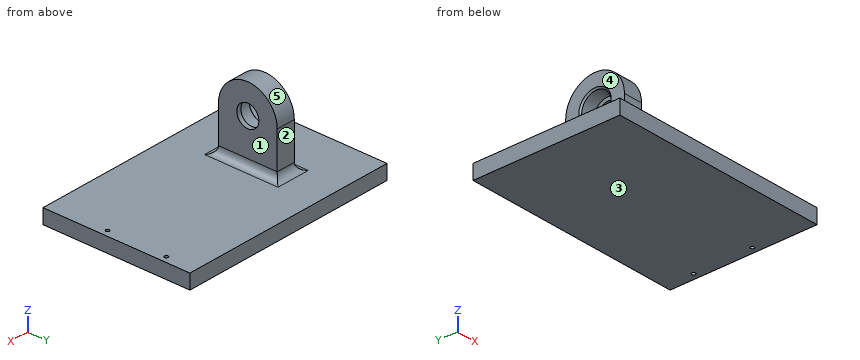
from build123d import *

# Parameters (mm, degrees)
SKETCH_2_W          = 150
SKETCH_2_H          = 100
EXTRUDE_1_DEPTH     = 10
SKETCH_3_W          = 13
SKETCH_3_H          = 40
EXTRUDE_2_DEPTH     = 40
SKETCH_4_R          = 20
EXTRUDE_3_DEPTH     = 13
SKETCH_5_R          = 10
CUT_EXTRUDE_1_DEPTH = 10
M3X0_5_2_D          = 2.5
FILLET_1_R          = 5
SKETCH_12_R         = 7.5
CUT_EXTRUDE_2_DEPTH = 130.263297188
CHAMFER_1_SIZE      = 1


with BuildPart() as part:
    # ｽｹｯﾁ2 → ﾎﾞｽ - 押し出し1 (new body)
    with BuildSketch(Plane.XY):
        Rectangle(SKETCH_2_W, SKETCH_2_H)
    extrude(amount=EXTRUDE_1_DEPTH)

    # ｽｹｯﾁ3 → ﾎﾞｽ - 押し出し2 (add)
    with BuildSketch(Plane.XY):
        with Locations((-31.5, 0)):
            Rectangle(SKETCH_3_W, SKETCH_3_H)
    extrude(amount=EXTRUDE_2_DEPTH)

    # ｽｹｯﾁ4 → ﾎﾞｽ - 押し出し3 (add)
    with BuildSketch(Plane.ZY.offset(38)):
        with Locations((40, 0)):
            Circle(SKETCH_4_R)
    extrude(amount=-EXTRUDE_3_DEPTH)

    # ｽｹｯﾁ5 → ｶｯﾄ - 押し出し1 (cut)
    with BuildSketch(Plane.ZY.offset(38)):
        with Locations(Location((40, 0, 0), (0, 0, 270))):
            Circle(SKETCH_5_R)
    extrude(amount=-CUT_EXTRUDE_1_DEPTH, mode=Mode.SUBTRACT)

    # M3x0.5 ねじ穴2 (through all)
    with Locations(Plane.XY.offset(10)):
        with Locations((70.5, -10.000898701), (70.5, 29.999101299)):
            Hole(M3X0_5_2_D / 2)

    # ﾌｨﾚｯﾄ1
    fillet_1_edges = [part.edges().sort_by_distance(p)[0] for p in [
        (-31.5, 20, 10),
        (-38, 0, 10),
        (-31.5, -20, 10),
        (-25, 0, 10),
    ]]
    fillet(fillet_1_edges, radius=FILLET_1_R)

    # ｽｹｯﾁ12 → ｶｯﾄ - 押し出し2 (cut, through all)
    with BuildSketch(Plane.ZY.offset(28)):
        with Locations(Location((40, 0, 0), (0, 0, 270))):
            Circle(SKETCH_12_R)
    extrude(amount=-CUT_EXTRUDE_2_DEPTH, mode=Mode.SUBTRACT)

    # 面取り1
    chamfer_1_edges = [part.edges().sort_by_distance(p)[0] for p in [
        (-38, 10, 40),
    ]]
    chamfer(chamfer_1_edges, length=CHAMFER_1_SIZE)


solid = part.part
Verification items for the finished model (mm, model axes). Face numbers are marked on the shaded views. A direction names the side the tool comes from. Coordinates: 2 decimals unless noted, no trailing zeros. Order: outer loops, then holes, each group sorted by start corner. A loop starts at its lowest first (then second) coordinate and runs counter-clockwise, first axis right, second up. Notation, with made-up numbers: M 50,76.5 L 78,76.5 A34 cw 78,113.5 Z; hole C 51.25,0.5 d6. An arc over 180 degrees is marked long. One line per item, written item: value. Start each with the question number.
Item 1: Scan lines: probe 1 along Y at (x, z) = (70, 3); probe 2 along Z at (x, y) = (26, 1); probe 3 along X at (y, z) = (-16, 18.5). Record each from-to range of solid material in increasing order.
Item 2: Sectioned sample at B-B (x = 4). Enter the section's corners in (y, z), then the cut area to 3 significant figures.
Item 3: Access from +Z, -Z, +X, -X, +Y, -Y to the whole of each face (thin tool, end or side, straight path). Record for the marked faces 1, 2, 3, 4 and 5.
Item 4: Gauge pin test, flat ends, axial feed: pin 1 (22 mm diameter, centred on y = 2, z = 43.5, fed in from -X); pin 2 (12 mm diameter, centred on x = 49.5, y = -5.5, fed in from +Z); pin 3 (4 mm diameter, centred on x = -34.5, z = 24.5, fed in from +Y); pin 4 (1 mm diameter, centred on x = -48.5, y = -13, fed in from -Z). Record the tip position at first contact, or that the pin passes through.
Item 5: Sectioned sample at C-C (y = 36). Enter the section's corners in (x, z), then the cut area to 3 significant figures.
Item 6: Sectioned sample at A-A (y = 0). Enter the section's corners in (x, z).
Conclusion:
1. probe 1: y = -50 to -11.15, -8.86 to 28.85, 31.14 to 50
1. probe 2: z = 0 to 10
1. probe 3: x = -38 to -25
2. outline: M -50,0 L 50,0 L 50,10 L -50,10 Z
2. area: 1,000 mm^2
3. face 1: +Z, +X, +Y, -Y
3. face 2: +Z, +X, -X, +Y
3. face 3: -Z, +X, -X, +Y, -Y
3. face 4: +Z, -X, +Y, -Y
3. face 5: +Z, +X, -X
4. pin 1: stops at x = -38
4. pin 2: stops at z = 10
4. pin 3: stops at y = 20
4. pin 4: stops at z = 0
5. outline: M -75,0 L 75,0 L 75,10 L -75,10 Z
5. area: 1,500 mm^2
6. outline: M -75,0 L 75,0 L 75,10 L -20,10 A5 cw -25,15 L -25,32.5 L -28,32.5 L -28,30 L -37,30 L -38,29 L -38,15 A5 cw -43,10 L -75,10 Z; M -38,51 L -37,50 L -28,50 L -28,47.5 L -25,47.5 L -25,60 L -38,60 Z
